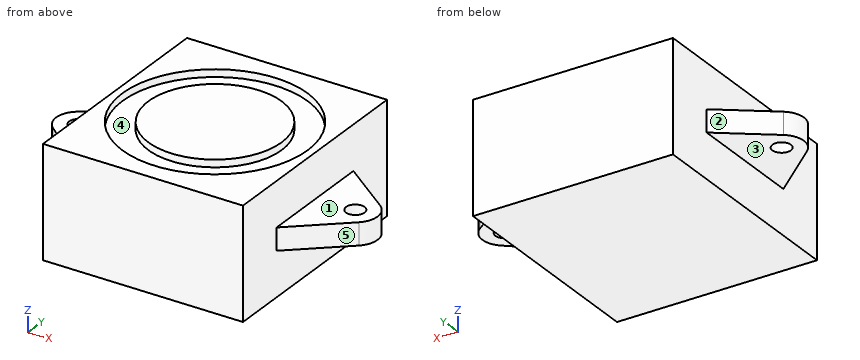
from build123d import *

# Parameters (mm, degrees)
SKETCH1_W           = 27
SKETCH1_H           = 30
BOSS_EXTRUDE1_DEPTH = 15
SKETCH2_R           = 12.5
SKETCH2_R_2         = 9
CUT_EXTRUDE1_DEPTH  = 1
SKETCH3_R           = 1.25
BOSS_EXTRUDE2_DEPTH = 9
SKETCH4_W           = 10.736601318
SKETCH4_H           = 16
CUT_EXTRUDE2_DEPTH  = 6


with BuildPart() as part:
    # Sketch1 → Boss-Extrude1 (new body)
    with BuildSketch(Plane.XY):
        with Locations((13.5, 15)):
            Rectangle(SKETCH1_W, SKETCH1_H)
    extrude(amount=BOSS_EXTRUDE1_DEPTH)

    # Sketch2 → Cut-Extrude1 (cut)
    with BuildSketch(Plane.XY.offset(15)):
        with Locations((13.5, 15)):
            Circle(SKETCH2_R)
        with Locations((13.5, 15)):
            Circle(SKETCH2_R_2, mode=Mode.SUBTRACT)
    extrude(amount=-CUT_EXTRUDE1_DEPTH, mode=Mode.SUBTRACT)

    # Sketch3 → Boss-Extrude2 (add)
    # profile 1 of 2: a face of its own
    with BuildSketch(Plane.XY.offset(15)):
        with BuildLine():
            Line((0, 7), (0, 23))
            Line((0, 23), (-6.989512345, 17.783175422))
            ThreePointArc((-6.989512345, 17.783175422), (-8.193484437, 15.477105093), (-7.142826585, 13.097267443))
            Line((-7.142826585, 13.097267443), (0, 7))
        make_face()
        with Locations((-5.195088865, 15.379003137)):
            Circle(SKETCH3_R, mode=Mode.SUBTRACT)
    # profile 2 of 2: a face of its own
    with BuildSketch(Plane.XY.offset(15)):
        with BuildLine():
            Line((27, 7), (34.142826585, 13.097267443))
            ThreePointArc((34.142826585, 13.097267443), (35.193484437, 15.477105093), (33.989512345, 17.783175422))
            Line((33.989512345, 17.783175422), (27, 23))
            Line((27, 23), (27, 7))
        make_face()
        with Locations((32.195088865, 15.379003137)):
            Circle(SKETCH3_R, mode=Mode.SUBTRACT)
    extrude(amount=-BOSS_EXTRUDE2_DEPTH)

    # Sketch4 → Cut-Extrude2 (cut)
    with BuildSketch(Plane.XY.offset(15)):
        Polygon((0, 23), (-13.068539103, 23), (-13.068539103, 5.328314146), (0, 7), align=None)
        with Locations((32.368300659, 15)):
            Rectangle(SKETCH4_W, SKETCH4_H)
    extrude(amount=-CUT_EXTRUDE2_DEPTH, mode=Mode.SUBTRACT)


solid = part.part
Design review of the part built by this model. Coordinates are the model's own, in mm. Face numbers are marked on the shaded views. A direction names the side the tool comes from. Coordinates: 2 decimals unless noted, no trailing zeros. Write each loop counter-clockwise with the first axis right and the second up, starting at its lowest first coordinate (ties: lowest second). Pieces come first, ordered by that corner, then holes. Notation, with made-up numbers: (50.5, 16.5) -> (79.5, 16.5) arc R19 cw to (79.5, 29.5) -> close; hole circle Ø6 at (36.25, 6.25). An arc over 180 degrees is marked (long way). Write each question's results on one line, items separated by ' | '. Start each with the question number.
(1) Tool access review of the marked faces 1 and 2: name each direction out of +Z, -Z, +X, -X, +Y, -Y from which nothing blocks a thin tool from reaching the whole face with its end or side.
(2) Take a section at A-A on x = 32. Write out the cut boundary in (y, z), and give its area (3 significant figures).
(3) Take a section at C-C on y = 12.5. Write out the cut boundary in (x, z), and give its area (3 significant figures).
(4) Take a section at B-B on x = 13.5. Write out the cut boundary in (y, z).
(5) Clearance check with flat-ended pins moving along their axes: P1, Ø4, axis at x = -5.2, y = 15.38, coming from the -Z side; P2, Ø4, axis at x = -4.5, y = 15, coming from the +Z side; P3, Ø6, axis at y = 9.5, z = 8.5, coming from the +X side; P4, Ø9, axis at x = 30.5, y = 18.5, coming from the +Z side. State where each tip first meets the part, or that it passes through.
(6) The part is to be moulded in two halves that separate along X. For the marked faces 3, 4 and 5, say which applies: pulls with the +X half, pulls with the -X half, needs draft (parallel to the pull), parting line crosses it, or undercut.
(7) For line 1 along X through (y, z) = (15.25, 7.5); line 2 along Y through (x, z) = (13.5, 14.3); line 3 along X through (y, z) = (24, 13.25), list the stretches that pass through material, from the lowest coordinate up. Write a range as from..to.
(8) Take a section at D-D on z = 9.75. Write out the cut boundary in (x, y), and give its area (3 significant figures).
Results found:
1) face 1: +Z, +X, +Y, -Y | face 2: +Z, -Z, -X, +Y
2) outline: (11.27, 6) -> (14.14, 6) -> (14.14, 9) -> (11.27, 9) -> close; (16.61, 6) -> (19.27, 6) -> (19.27, 9) -> (16.61, 9) -> close | area: 16.6 mm2
3) outline: (-6.44, 6) -> (0, 6) -> (0, 0) -> (27, 0) -> (27, 6) -> (33.44, 6) -> (33.44, 9) -> (27, 9) -> (27, 15) -> (25.75, 15) -> (25.75, 14) -> (22.15, 14) -> (22.15, 15) -> (4.85, 15) -> (4.85, 14) -> (1.25, 14) -> (1.25, 15) -> (0, 15) -> (0, 9) -> (-6.44, 9) -> close | area: 436 mm2
4) outline: (0, 0) -> (30, 0) -> (30, 15) -> (27.5, 15) -> (27.5, 14) -> (24, 14) -> (24, 15) -> (6, 15) -> (6, 14) -> (2.5, 14) -> (2.5, 15) -> (0, 15) -> close
5) P1: stops at z = 6 | P2: stops at z = 9 | P3: stops at x = 33.44 | P4: stops at z = 15
6) face 3: needs draft | face 4: undercut | face 5: pulls with the +X half
7) line 1: x = -8.19..-6.44, -3.95..30.95, 33.44..35.19 | line 2: y = 0..2.5, 6..24, 27.5..30 | line 3: x = 0..27
8) outline: (0, 0) -> (27, 0) -> (27, 30) -> (0, 30) -> close | area: 810 mm2
